Can you work these out from the drawing? Everything is in mm from the part's minimum corner. A direction names the side the tool comes from. Round coordinates to 2 decimals unless told otherwise and drop trailing zeros. Write each loop counter-clockwise with the first axis right and the second up, starting at its lowest first coordinate (ties: lowest second). Pieces come first, ordered by that corner, then holes. Notation, with made-up numbers: (-14.75, 45) -> (-7.75, 45) arc R26 ccw to (-7.75, 71) -> close; hole circle Ø4 at (-32, 76). An arc over 180 degrees is marked (long way). Put each result on its own line as item: value. Start each with the question number.
1. Which directions (+Z, -Z, +X, -X, +Y, -Y) give clear straight access to the entire face, cutting with the end or side of a thin tool? Please do the marked faces 5, 6 and 7.
2. For pin 1 (1 mm diameter, centred on y = 24.5, z = 9.5, fed in from -X); pin 2 (13.5 mm diameter, centred on x = 9, z = 15, fed in from +Y), each with a flat end and sliding along its axis, tell me the tip position at first contact or that it passes through.
3. Suppose I cut it at A-A (x = 35). Please give me the cut outline in (y, z).
4. Suppose I cut it at C-C (y = 32). Please give me the cut outline in (x, z) (3 decimals).
5. Suppose I cut it at D-D (y = 14.5). Please give me the cut outline in (x, z), then the cut area to 3 significant figures.
6. I need wall thicknesses on probe 1 along Y at (x, z) = (35, 21.3); probe 2 along X at (y, z) = (20.5, 12); probe 3 along Z at (x, y) = (9, 6). Which ranges of each line are inside material? Lowest first, please. Write a range as from..to.
7. Suppose I cut it at B-B (z = 12). Please give me the cut outline in (x, y).
8. We'd pull the mould along Y, two halves only. Please class the marked faces 1, 2, 3 and 4: +Y half, -Y half, draft (parallel to the pull), parting line (faces both ways), or undercut.
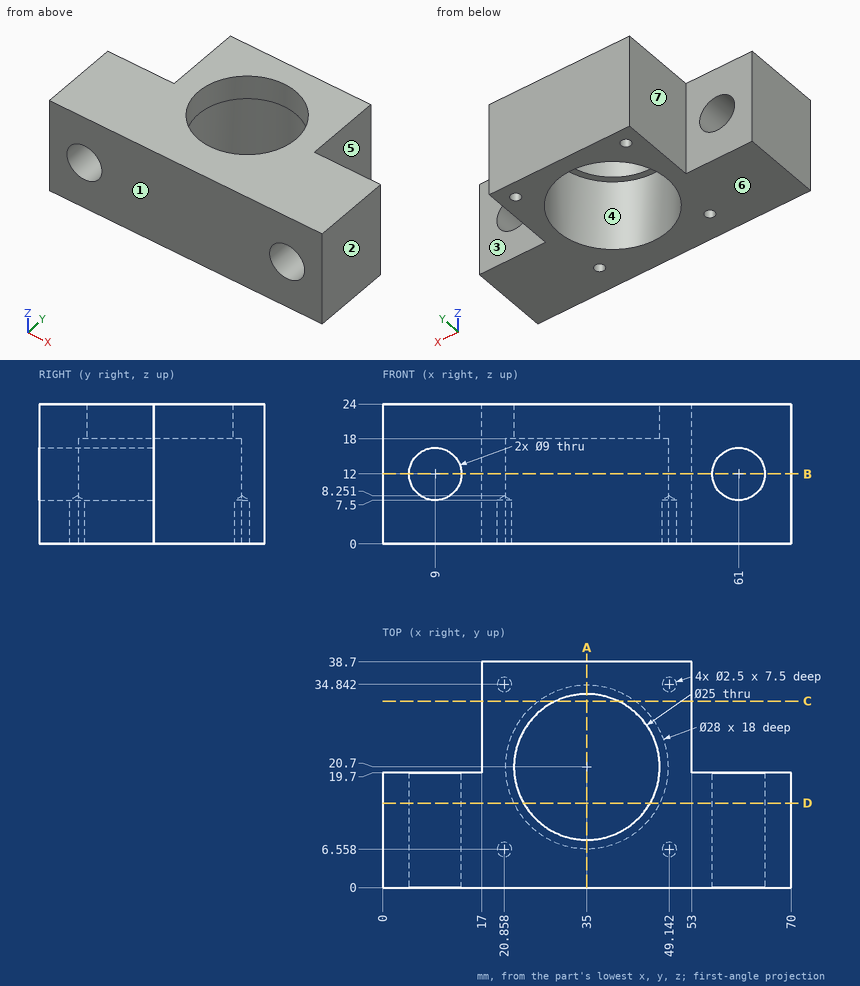
Verdict:
1. face 5: +Z, -Z, +X, +Y
1. face 6: -Z, +X, -X, +Y, -Y
1. face 7: +Z, -Z, -X, +Y
2. pin 1: stops at x = 17
2. pin 2: stops at y = 19.7
3. outline: (0, 0) -> (6.7, 0) -> (6.7, 18) -> (8.2, 18) -> (8.2, 24) -> (0, 24) -> close; (33.2, 18) -> (34.7, 18) -> (34.7, 0) -> (38.7, 0) -> (38.7, 24) -> (33.2, 24) -> close
4. outline: (17, 0) -> (26.735, 0) -> (26.735, 18) -> (29.656, 18) -> (29.656, 24) -> (17, 24) -> close; (40.344, 18) -> (43.265, 18) -> (43.265, 0) -> (53, 0) -> (53, 24) -> (40.344, 24) -> close
5. outline: (0, 0) -> (22.45, 0) -> (22.45, 18) -> (24.15, 18) -> (24.15, 24) -> (0, 24) -> close; (45.85, 18) -> (47.55, 18) -> (47.55, 0) -> (70, 0) -> (70, 24) -> (45.85, 24) -> close; hole circle Ø9 at (9, 12); hole circle Ø9 at (61, 12)
5. area: 971 mm^2
6. probe 1: y = 0..8.2, 33.2..38.7
6. probe 2: x = 17..21, 49..53
6. probe 3: z = 0..7.5, 16.5..24
7. outline: (0, 0) -> (4.5, 0) -> (4.5, 19.7) -> (0, 19.7) -> close; (13.5, 0) -> (56.5, 0) -> (56.5, 19.7) -> (53, 19.7) -> (53, 38.7) -> (17, 38.7) -> (17, 19.7) -> (13.5, 19.7) -> close; (65.5, 0) -> (70, 0) -> (70, 19.7) -> (65.5, 19.7) -> close; hole circle Ø28 at (35, 20.7)
8. face 1: -Y half
8. face 2: draft
8. face 3: +Y half
8. face 4: undercut
